```python
from build123d import *

# Parameters (mm, degrees)
F0_W     = 50.8
F0_H     = 50.8
F1_DEPTH = 12.7
F2_W     = 38.1
F2_H     = 38.1
F3_DEPTH = 152.4
F4_R     = 5.08
F5_R     = 3.175


with BuildPart() as f1:
    # F0 (on Top) → F1 (new body)
    with BuildSketch(Plane.XY):
        with Locations((-25.4, 25.4)):
            Rectangle(F0_W, F0_H)
    extrude(amount=F1_DEPTH)

    # F2 (on face) → F3 (join)
    with BuildSketch(Plane.XY.offset(12.7)):
        with Locations((-25.4, 25.4)):
            Rectangle(F2_W, F2_H)
    extrude(amount=F3_DEPTH)

    # F4
    f4_edges = [f1.edges().sort_by_distance(p)[0] for p in [
        (-25.4, 6.35, 12.7),
        (-6.35, 25.4, 12.7),
        (-25.4, 44.45, 12.7),
        (-44.45, 25.4, 12.7),
        (-44.45, 44.45, 88.9),
        (-44.45, 6.35, 88.9),
        (-6.35, 6.35, 88.9),
        (-6.35, 44.45, 88.9),
    ]]
    fillet(f4_edges, radius=F4_R)

    # F5
    f5_edges = [f1.edges().sort_by_distance(p)[0] for p in [
        (-25.4, 0, 0),
        (0, 25.4, 0),
        (-25.4, 50.8, 0),
        (-50.8, 25.4, 0),
    ]]
    fillet(f5_edges, radius=F5_R)


solid = f1.part
```
The model under review builds one solid part; all positions refer to its coordinate system, in mm. A direction names the side the tool comes from. Round coordinates to 2 decimals unless told otherwise and drop trailing zeros. Order: outer loops, then holes, each group sorted by start corner. A loop starts at its lowest first (then second) coordinate and runs counter-clockwise, first axis right, second up.
Item 1: To check wall thickness, follow probe 1 along X at (y, z) = (32, 47); probe 2 along Y at (x, z) = (-33, 99.5); probe 3 along Y at (x, z) = (-42, 64.5). State the ranges of each line that lie inside material, in increasing order.
Working result:
probe 1: x = -44.45 to -6.35
probe 2: y = 6.35 to 44.45
probe 3: y = 7.08 to 43.72
Item 2: Add section A-A, the plane x = -14. State the section outline as (y, z) points (3 decimals), and give its area (3 significant figures).
Working result:
outline: (0, 3.175) arc R3.175 ccw to (3.175, 0) - (47.625, 0) arc R3.175 ccw to (50.8, 3.175) - (50.8, 12.7) - (49.53, 12.7) arc R5.08 cw to (44.45, 17.78) - (44.45, 165.1) - (6.35, 165.1) - (6.35, 17.78) arc R5.08 cw to (1.27, 12.7) - (0, 12.7) - close
area: 6,460 mm2
Item 3: Machinability: for faces 1 (the flat face through (-27, 1, 12.7)), 2 (the cylindrical face through (-7.799, 42.922, 92.471)), 3 (the cylindrical face through (-7.878, 7.799, 92.471)), 4 (the cylindrical face through (-42.922, 7.799, 92.471)), which of the approach directions +Z, -Z, +X, -X, +Y, -Y give a long, thin tool a straight path to every point of the face, cutting with its end or side? Answer none if there is none.
Working result:
face 1: +Z
face 2: +Z, +X, +Y
face 3: +Z, +X, -Y
face 4: +Z, -X, -Y
Item 4: Add section C-C, the plane y = 18.5. State the section outline as (x, z) points (3 decimals), and give its area (3 significant figures).
Working result:
outline: (-50.8, 3.175) arc R3.175 ccw to (-47.625, 0) - (-3.175, 0) arc R3.175 ccw to (0, 3.175) - (0, 12.7) - (-1.27, 12.7) arc R5.08 cw to (-6.35, 17.78) - (-6.35, 165.1) - (-44.45, 165.1) - (-44.45, 17.78) arc R5.08 cw to (-49.53, 12.7) - (-50.8, 12.7) - close
area: 6,460 mm2
Item 5: For pin 1 (8.5 mm diameter, centred on x = -24.5, z = 88, fed in from +Y); pin 2 (8.5 mm diameter, centred on x = -30, z = 93, fed in from -Y); pin 3 (12 mm diameter, centred on y = 39.5, z = 21, fed in from -X), all flat-tipped, find the tip position at first contact; note any pin that passes through.
Working result:
pin 1: stops at y = 44.45
pin 2: stops at y = 6.35
pin 3: stops at x = -45.28
Item 6: Add section B-B, the plane z = 62. State the section outline as (x, y) points.
Working result:
outline: (-44.45, 11.43) arc R5.08 ccw to (-39.37, 6.35) - (-11.43, 6.35) arc R5.08 ccw to (-6.35, 11.43) - (-6.35, 39.37) arc R5.08 ccw to (-11.43, 44.45) - (-39.37, 44.45) arc R5.08 ccw to (-44.45, 39.37) - close
